from build123d import *

# Parameters (mm, degrees)
SKETCH_1_W      = 17.7
SKETCH_1_H      = 17.7
EXTRUDE_1_DEPTH = 8.7
SKETCH_2_R      = 7.35
EXTRUDE_2_DEPTH = 21.8
SKETCH_3_W      = 3
SKETCH_3_H      = 0.3
EXTRUDE_3_DEPTH = 6.8
FILLET_1_R      = 0.8
SKETCH_4_W      = 17
SKETCH_4_H      = 17
EXTRUDE_4_DEPTH = 1
CHAMFER_1_SIZE  = 0.2


with BuildPart() as part:
    # 草图1 → 凸台-拉伸1 (new body)
    with BuildSketch(Plane(origin=(0, 0, 0), x_dir=(1, 0, 0), z_dir=(0, 1, 0))):
        Rectangle(SKETCH_1_W, SKETCH_1_H)
    extrude(amount=EXTRUDE_1_DEPTH)

    # 草图2 → 凸台-拉伸2 (add)
    with BuildSketch(Plane.XZ):
        Circle(SKETCH_2_R)
    extrude(amount=EXTRUDE_2_DEPTH)

    # 草图3 → 凸台-拉伸3 (add)
    with BuildSketch(Plane.XZ.offset(21.8)):
        with Locations((-5, -1.65)):
            Rectangle(SKETCH_3_W, SKETCH_3_H)
        with Locations((0, -1.65)):
            Rectangle(SKETCH_3_W, SKETCH_3_H)
        with Locations((5, -1.65)):
            Rectangle(SKETCH_3_W, SKETCH_3_H)
    extrude(amount=EXTRUDE_3_DEPTH)

    # 圆角1
    fillet_1_edges = [part.edges().sort_by_distance(p)[0] for p in [
        (-6.5, -28.6, -1.65),
        (-3.5, -28.6, -1.65),
        (-1.5, -28.6, -1.65),
        (1.5, -28.6, -1.65),
        (3.5, -28.6, -1.65),
        (6.5, -28.6, -1.65),
    ]]
    fillet(fillet_1_edges, radius=FILLET_1_R)

    # 草图4 → 凸台-拉伸4 (add)
    with BuildSketch(Plane(origin=(0, 8.7, 0), x_dir=(1, 0, 0), z_dir=(0, 1, 0))):
        Rectangle(SKETCH_4_W, SKETCH_4_H)
    extrude(amount=EXTRUDE_4_DEPTH)

    # 倒角1
    chamfer_1_edges = [part.edges().sort_by_distance(p)[0] for p in [
        (-8.85, 8.7, 0),
        (0, 8.7, 8.85),
        (8.85, 8.7, 0),
        (0, 8.7, -8.85),
    ]]
    chamfer(chamfer_1_edges, length=CHAMFER_1_SIZE)


solid = part.part
Build history of the part. All positions in model axes, mm. A direction names the side the tool comes from. Round coordinates to 2 decimals unless told otherwise and drop trailing zeros. Order: outer loops, then holes, each group sorted by start corner. A loop starts at its lowest first (then second) coordinate and runs counter-clockwise, first axis right, second up. Notation, with made-up numbers: M 57,65.25 L 90,65.25 A15 ccw 90,83.25 Z; hole C -31.5,-37 d10. An arc over 180 degrees is marked long. Use CSV: the item, a comma, the result in double quotes. Start each with the question number.
(1) Cut at B-B on z = 0. List the corners of the cut face in (x, y), then the cut area to 3 significant figures.
(2) Cut at D-D on y = -20. List the corners of the cut face in (x, z).
(3) Flat gauge pins, fed straight in: P1, Ø8, axis at y = -14, z = 5, coming from the +X side; P2, Ø0.5, axis at y = 9.5, z = -3, coming from the -X side; P3, Ø0.8, axis at x = -2, y = 9, coming from the -Z side. Where does each tip first touch, or does it go through?
(4) Tool access for faces 1 (the face through (-5, -25, -1.8)), 2 (the face through (8.5, 9, 0)), 3 (the face through (0, -25, -1.5)), 4 (the face through (-8.5, 9, 0)): list every direction of +Z, -Z, +X, -X, +Y, -Y with a clear straight run to the whole face (end or side of a thin tool).
(5) Drill centre lines: probe 1 along Y at (x, z) = (-1.5, -2.75); probe 2 along Y at (x, z) = (-7.5, -6); probe 3 along Z at (x, y) = (-5.5, -23). Where is each one in solid material? Low to high.
(6) Cut at C-C on x = 3. List the corners of the cut face in (y, z).
(7) Cut at A-A on y = -25.5. List the corners of the cut face in (x, z).
Findings:
1,outline,"M -8.85,0 L -7.35,0 L -7.35,-21.8 L 7.35,-21.8 L 7.35,0 L 8.85,0 L 8.85,8.5 L 8.65,8.7 L 8.5,8.7 L 8.5,9.7 L -8.5,9.7 L -8.5,8.7 L -8.65,8.7 L -8.85,8.5 Z"
1,area,"491 mm^2"
2,outline,"C 0,0 d14.7"
3,P1,"stops at x = 7.28"
3,P2,"stops at x = -8.5"
3,P3,"stops at z = -8.75"
4,face 1,"-Z, +X, -X, -Y"
4,face 2,"+Z, -Z, +X, +Y"
4,face 3,"+Z, +X, -X, -Y"
4,face 4,"+Z, -Z, -X, +Y"
5,probe 1,"y = -21.8 to 9.7"
5,probe 2,"y = 0 to 9.7"
5,probe 3,"z = -1.8 to -1.5"
6,outline,"M -21.8,-6.71 L 0,-6.71 L 0,-8.85 L 8.5,-8.85 L 8.7,-8.65 L 8.7,-8.5 L 9.7,-8.5 L 9.7,8.5 L 8.7,8.5 L 8.7,8.65 L 8.5,8.85 L 0,8.85 L 0,6.71 L -21.8,6.71 Z"
7,outline,"M -6.5,-1.8 L -3.5,-1.8 L -3.5,-1.5 L -6.5,-1.5 Z; M -1.5,-1.8 L 1.5,-1.8 L 1.5,-1.5 L -1.5,-1.5 Z; M 3.5,-1.8 L 6.5,-1.8 L 6.5,-1.5 L 3.5,-1.5 Z"
